CAD build for the part. Positions are in the model's coordinates, mm. A direction names the side the tool comes from. Coordinates: 2 decimals unless noted, no trailing zeros. Order: outer loops, then holes, each group sorted by start corner. A loop starts at its lowest first (then second) coordinate and runs counter-clockwise, first axis right, second up. Notation, with made-up numbers: M -9.5,-11.5 L 20.5,-11.5 A29 ccw 20.5,12.5 Z; hole C 61,-26 d1. An arc over 180 degrees is marked long. Write item = value, one per line.
from build123d import *

# Parameters (mm, degrees)
DODANIE_WYCI_GNI_CIE1_DEPTH = 5
DODANIE_WYCI_GNI_CIE2_START = -5
SZKIC2_R                    = 6
DODANIE_WYCI_GNI_CIE2_DEPTH = 5
WYTNIJ_WYCI_GNI_CIE1_DEPTH  = 716.158788588


with BuildPart() as part:
    # Szkic1 → Dodanie-wyciągnięcie1 (new body)
    with BuildSketch(Plane.XY):
        with BuildLine():
            ThreePointArc((-241.458717663, 517.809891046), (0, 571.34), (241.458717663, 517.809891046))
            Line((241.458717663, 517.809891046), (275.268178602, 590.314514008))
            ThreePointArc((275.268178602, 590.314514008), (0, 651.34), (-275.268178602, 590.314514008))
            Line((-275.268178602, 590.314514008), (-241.458717663, 517.809891046))
        make_face()
        with BuildLine():
            ThreePointArc((-220.327804576, 472.494501694), (0, 521.34), (220.327804576, 472.494501694))
            Line((220.327804576, 472.494501694), (241.458717663, 517.809891046))
            ThreePointArc((241.458717663, 517.809891046), (0, 571.34), (-241.458717663, 517.809891046))
            Line((-241.458717663, 517.809891046), (-220.327804576, 472.494501694))
        make_face()
    extrude(amount=DODANIE_WYCI_GNI_CIE1_DEPTH)

    # Szkic2 → Dodanie-wyciągnięcie2 (add)
    with BuildSketch(Plane.XY.offset(5).offset(DODANIE_WYCI_GNI_CIE2_START)):
        with BuildLine():
            Line((-293.394334343, 581.862148774), (-238.453960317, 464.042136459))
            ThreePointArc((-238.453960317, 464.042136459), (-212.049678092, 454.288112103), (-202.042855969, 480.597627909))
            ThreePointArc((-202.042855969, 480.597627909), (0, 521.34), (202.042855969, 480.597627909))
            ThreePointArc((202.042855969, 480.597627909), (212.049678092, 454.288112103), (238.453960317, 464.042136459))
            Line((238.453960317, 464.042136459), (293.394334343, 581.862148774))
            ThreePointArc((293.394334343, 581.862148774), (283.581145562, 608.505021982), (257.014390413, 598.487592788))
            ThreePointArc((257.014390413, 598.487592788), (0, 651.34), (-257.014390413, 598.487592788))
            ThreePointArc((-257.014390413, 598.487592788), (-283.581145562, 608.505021982), (-293.394334343, 581.862148774))
        make_face()
        with Locations((-279.424662082, 599.409767995)):
            Circle(SZKIC2_R, mode=Mode.SUBTRACT)
        with Locations((-216.188741334, 463.391306898)):
            Circle(SZKIC2_R, mode=Mode.SUBTRACT)
        with Locations((216.188741334, 463.391306898)):
            Circle(SZKIC2_R, mode=Mode.SUBTRACT)
        with Locations((279.424662082, 599.409767995)):
            Circle(SZKIC2_R, mode=Mode.SUBTRACT)
    extrude(amount=DODANIE_WYCI_GNI_CIE2_DEPTH)

    # Szkic4 → Wytnij-wyciągnięcie1 (cut, through all)
    with BuildSketch(Plane.XY.offset(5)):
        with BuildLine():
            ThreePointArc((234.78479941, 515.380532778), (238.578545987, 515.23612037), (241.380121814, 517.798256378))
            Line((241.380121814, 517.798256378), (241.398609626, 517.837915637))
            ThreePointArc((241.398609626, 517.837915637), (241.544560472, 521.672077329), (238.930450422, 524.480729352))
            ThreePointArc((238.930450422, 524.480729352), (0, 576.34), (-238.930450422, 524.480729352))
            ThreePointArc((-238.930450422, 524.480729352), (-241.544560472, 521.672077329), (-241.398609626, 517.837915637))
            Line((-241.398609626, 517.837915637), (-241.380121814, 517.798256378))
            ThreePointArc((-241.380121814, 517.798256378), (-238.578545987, 515.23612037), (-234.78479941, 515.380532778))
            ThreePointArc((-234.78479941, 515.380532778), (0, 566.34), (234.78479941, 515.380532778))
        make_face()
    extrude(amount=-WYTNIJ_WYCI_GNI_CIE1_DEPTH, mode=Mode.SUBTRACT)


solid = part.part
(1) Slice it at D-D, the plane z = 3.7. Write the cut outline in (x, y).
Evaluation:
outline = M -293.39,581.86 L -238.45,464.04 A20 ccw -202.04,480.6 A521.34 cw 202.04,480.6 A20 ccw 238.45,464.04 L 293.39,581.86 A20 ccw long 257.01,598.49 A651.34 ccw -257.01,598.49 A20 ccw long Z; hole C -279.42,599.41 d12; hole M -241.4,517.84 L -241.38,517.8 A5 ccw -234.78,515.38 A566.34 cw 234.78,515.38 A5 ccw 241.38,517.8 L 241.4,517.84 A5 ccw 238.93,524.48 A576.34 ccw -238.93,524.48 A5 ccw Z; hole C -216.19,463.39 d12; hole C 216.19,463.39 d12; hole C 279.42,599.41 d12
(2) Pin check, flat tip, straight feed: pin 1 Ø1.5 at (y, z) = (498.5, 4) entering from +X. Stop position of the tip, or through.
Evaluation:
pin_1 = 254.87
(3) Slice it at B-B, the plane y = 547. Write the cut outline in (x, z), then the cut area to 3 significant figures.
Evaluation:
outline = M -277.14,0 L -181.55,0 L -181.55,5 L -277.14,5 Z; M -146.74,0 L 146.74,0 L 146.74,5 L -146.74,5 Z; M 181.55,0 L 277.14,0 L 277.14,5 L 181.55,5 Z
area = 2,420 mm²
(4) Wall check: line 1 (X direction, y = 526, z = 2); line 2 (Y direction, x = 215.5, z = 1.8); line 3 (X direction, y = 597.5, z = 3.5). Give the ranges that are in metal, low to high. Write a range as from..to.
Evaluation:
line_1 = -267.35..-235.57, -209.92..209.92, 235.57..267.35
line_2 = 453.09..457.43, 469.35..523.74, 534.53..614.66
line_3 = -293.93..-285.11, -273.74..273.74, 285.11..293.93
(5) Slice it at C-C, the plane y = 487.5. Write the cut outline in (x, z).
Evaluation:
outline = M -249.39,0 L -184.77,0 L -184.77,5 L -249.39,5 Z; M 184.77,0 L 249.39,0 L 249.39,5 L 184.77,5 Z
(6) Tool access for faces 1 (the face through (3.45, 576.33, 2.54)), 2 (the face through (265.54, 522.13, 2.46)): list every direction of +Z, -Z, +X, -X, +Y, -Y with a clear straight run to the whole face (end or side of a thin tool).
Evaluation:
face_1 = +Z, -Z
face_2 = +Z, -Z, +X, -Y
(7) Slice it at A-A, the plane x = -183. Write the cut outline in (y, z), then the cut area to 3 significant figures.
Evaluation:
outline = M 488.17,0 L 535.96,0 L 535.96,5 L 488.17,5 Z; M 546.52,0 L 625.1,0 L 625.1,5 L 546.52,5 Z
area = 632 mm²
(8) Pull direction X, two halves, no side cores. Call faces 3 (the face through (-266.31, 523.78, 2.46)), 4 (the face through (218.96, 458.07, 2.46)), 5 (the face through (-4, 553, 0)): +X half, -X half, draft (parallel to the pull), parting line (faces both ways), or undercut.
Evaluation:
face_3 = -X half
face_4 = undercut
face_5 = draft
